from build123d import *

# Parameters (mm, degrees)
SKETCH001_W   = 78
SKETCH001_H   = 5
PAD001_DEPTH  = 60
SKETCH_W      = 2
SKETCH_H      = 30
PAD_DEPTH     = 60
ARRAY_X_COUNT = 7
ARRAY_X_PITCH = 11.25


with BuildPart() as pad001:
    # Sketch001 → Pad001 (new body)
    with BuildSketch(Plane.XY):
        with Locations((0, -2.5)):
            Rectangle(SKETCH001_W, SKETCH001_H)
    extrude(amount=PAD001_DEPTH)


with BuildPart() as fusion:
    # Sketch → Pad (new body)
    with BuildSketch(Plane.XY):
        with Locations((-34, -20)):
            Rectangle(SKETCH_W, SKETCH_H)
    extrude(amount=PAD_DEPTH)

    # Array X: Fusion ×7


with BuildPart() as fusion_1:
    add(fusion.part)
    with Locations(*[(i * ARRAY_X_PITCH, 0, 0) for i in range(1, ARRAY_X_COUNT)]):
        add(fusion.part)

    # Fusion: union Pad001
    add(pad001.part)


solid = fusion_1.part
Can you work these out from the model? Positions are in its coordinate system, mm. A direction names the side the tool comes from. Round coordinates to 2 decimals unless told otherwise and drop trailing zeros. Order: outer loops, then holes, each group sorted by start corner. A loop starts at its lowest first (then second) coordinate and runs counter-clockwise, first axis right, second up. Notation, with made-up numbers: M -19,42.5 L 3,42.5 A23 ccw 3,55.5 Z; hole C 27.5,87 d5. An arc over 180 degrees is marked long. Use a Markdown table: item, result.
1) I'm going to push flat-ended pins straight in: P1, Ø15, axis at y = -14, z = 19, coming from the -X side; P2, Ø1.2, axis at x = -36, z = 18.5, coming from the -Y side. Where does each tip first touch, or does it pass through?
Geometry says:
| item | result |
|---|---|
| P1 | stops at x = -35 |
| P2 | stops at y = -5 |
2) Imagine slicing it at C-C (x = -5). List the corners of the cut face in (y, z) for me.
Geometry says:
| item | result |
|---|---|
| outline | M -5,0 L 0,0 L 0,60 L -5,60 Z |
3) If we mould it in two halves opening along X, with no side actions, what happens to faces 4 (the face through (39, -3, 30)), 5 (the face through (-37, -5, 30)), 6 (the face through (12, -20, 30))? For each: +X half, -X half, draft (parallel to the pull), parting line (faces both ways), or undercut.
Geometry says:
| item | result |
|---|---|
| face 4 | +X half |
| face 5 | draft |
| face 6 | undercut |
4) Imagine slicing it at A-A (y = -23). List the corners of the cut face in (x, z) for me.
Geometry says:
| item | result |
|---|---|
| outline | M -35,0 L -33,0 L -33,60 L -35,60 Z; M -23.75,0 L -21.75,0 L -21.75,60 L -23.75,60 Z; M -12.5,0 L -10.5,0 L -10.5,60 L -12.5,60 Z; M -1.25,0 L 0.75,0 L 0.75,60 L -1.25,60 Z; M 10,0 L 12,0 L 12,60 L 10,60 Z; M 21.25,0 L 23.25,0 L 23.25,60 L 21.25,60 Z; M 32.5,0 L 34.5,0 L 34.5,60 L 32.5,60 Z |
5) On a 3-axis mill with a long thin cutter (end or side, diameter ignored), from which of +Z, -Z, +X, -X, +Y, -Y can I reach the whole of each face in a straight line? I mean faces 1 (the face through (22, -35, 30)), 2 (the face through (34.5, -20, 30)), 3 (the face through (-33, -20, 30)). Say none if no direction works.
Geometry says:
| item | result |
|---|---|
| face 1 | +Z, -Z, +X, -X, -Y |
| face 2 | +Z, -Z, +X, -Y |
| face 3 | +Z, -Z, -Y |
6) If I drill on line 1 along Y through (x, z) = (28.5, 9), over which ranges is the centre line in solid material (lowest first)?
Geometry says:
| item | result |
|---|---|
| line 1 | y = -5 to 0 |
